from build123d import *

# Parameters (mm, degrees)
ESBO_O2_W                = 30
ESBO_O2_H                = 70
RESSALTO_EXTRUS_O1_DEPTH = 8
ESBO_O3_R                = 0.75
CORTE_EXTRUS_O1_DEPTH    = 30
FILETE1_R                = 2
ESBO_O17_W               = 10
ESBO_O17_H               = 5
RESSALTO_EXTRUS_O4_DEPTH = 8
ESBO_O20_R               = 2
CORTE_EXTRUS_O9_DEPTH    = 8
FILETE2_R                = 2.5
FILETE3_R                = 2.5
FILETE4_R                = 2.5
FILETE5_R                = 2.5
ESBO_O21_W               = 5
ESBO_O21_H               = 20
CORTE_EXTRUS_O10_DEPTH   = 9
FILETE6_R                = 2.5
ESBO_O22_R               = 1.5
CORTE_EXTRUS_O11_DEPTH   = 20
ESBO_O23_R               = 1.75
CORTE_EXTRUS_O12_DEPTH   = 22


with BuildPart() as part:
    # Esboço2 → Ressalto-extrusão1 (new body)
    with BuildSketch(Plane.XY):
        with Locations((-52.281248797, -0.107598663)):
            Rectangle(ESBO_O2_W, ESBO_O2_H)
    extrude(amount=RESSALTO_EXTRUS_O1_DEPTH)

    # Esboço3 → Corte-extrusão1 (cut)
    with BuildSketch(Plane(origin=(0, -35.107598663, 0), x_dir=(-1, 0, 0), z_dir=(0, -1, 0))):
        with Locations((58.281248797, -4)):
            Circle(ESBO_O3_R)
        with Locations((63.281248797, -4)):
            Circle(ESBO_O3_R)
    extrude(amount=-CORTE_EXTRUS_O1_DEPTH, mode=Mode.SUBTRACT)

    # Filete1
    filete1_edges = [part.edges().sort_by_distance(p)[0] for p in [
        (-37.281248797, -0.107598663, 8),
    ]]
    fillet(filete1_edges, radius=FILETE1_R)

    # Esboço17 → Ressalto-extrusão4 (add)
    with BuildSketch(Plane(origin=(0, 0, 0), x_dir=(-1, 0, 0), z_dir=(0, 0, -1))):
        with Locations((72.281248797, -32.607598663)):
            Rectangle(ESBO_O17_W, ESBO_O17_H)
    extrude(amount=-RESSALTO_EXTRUS_O4_DEPTH)

    # Esboço20 → Corte-extrusão9 (cut)
    with BuildSketch(Plane.XZ.offset(35.107598663)):
        with Locations((-73.951248797, 4)):
            Circle(ESBO_O20_R)
    extrude(amount=-CORTE_EXTRUS_O9_DEPTH, mode=Mode.SUBTRACT)

    # Filete2
    filete2_edges = [part.edges().sort_by_distance(p)[0] for p in [
        (-67.281248797, 2.392401337, 8),
    ]]
    fillet(filete2_edges, radius=FILETE2_R)

    # Filete3
    filete3_edges = [part.edges().sort_by_distance(p)[0] for p in [
        (-67.281248797, 2.392401337, 0),
    ]]
    fillet(filete3_edges, radius=FILETE3_R)

    # Filete4
    filete4_edges = [part.edges().sort_by_distance(p)[0] for p in [
        (-77.281248797, -32.607598663, 8),
    ]]
    fillet(filete4_edges, radius=FILETE4_R)

    # Filete5
    filete5_edges = [part.edges().sort_by_distance(p)[0] for p in [
        (-77.281248797, -32.607598663, 0),
    ]]
    fillet(filete5_edges, radius=FILETE5_R)

    # Esboço21 → Corte-extrusão10 (cut, through all)
    with BuildSketch(Plane.XY.offset(8)):
        with Locations((-44.781248797, 18.892401337)):
            Rectangle(ESBO_O21_W, ESBO_O21_H)
        with Locations((-44.781248797, -19.107598663)):
            Rectangle(ESBO_O21_W, ESBO_O21_H)
    extrude(amount=-CORTE_EXTRUS_O10_DEPTH, mode=Mode.SUBTRACT)

    # Filete6
    filete6_edges = [part.edges().sort_by_distance(p)[0] for p in [
        (-37.281248797, -0.107598663, 0),
    ]]
    fillet(filete6_edges, radius=FILETE6_R)

    # Esboço22 → Corte-extrusão11 (cut)
    with BuildSketch(Plane(origin=(-37.281248797, 0, 0), x_dir=(0, 0, -1), z_dir=(1, 0, 0))):
        with Locations((-5, -25.107598663)):
            Circle(ESBO_O22_R)
        with Locations((-5, -14.107598663)):
            Circle(ESBO_O22_R)
        with Locations((-5, 24.892401337)):
            Circle(ESBO_O22_R)
        with Locations((-5, 13.892401337)):
            Circle(ESBO_O22_R)
    extrude(amount=-CORTE_EXTRUS_O11_DEPTH, mode=Mode.SUBTRACT)

    # Esboço23 → Corte-extrusão12 (cut)
    with BuildSketch(Plane(origin=(0, 34.892401337, 0), x_dir=(1, 0, 0), z_dir=(0, 1, 0))):
        with Locations((-62.281248797, -4)):
            Circle(ESBO_O23_R)
    extrude(amount=-CORTE_EXTRUS_O12_DEPTH, mode=Mode.SUBTRACT)


solid = part.part
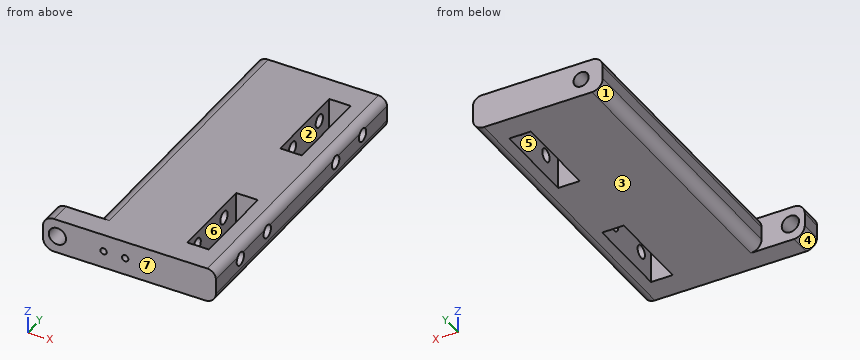
Read the model definition and answer for the solid it produces. Units are mm, in the model's axes. Face numbers are marked on the shaded views. A direction names the side the tool comes from. Round coordinates to 2 decimals unless told otherwise and drop trailing zeros. Order: outer loops, then holes, each group sorted by start corner. A loop starts at its lowest first (then second) coordinate and runs counter-clockwise, first axis right, second up. Notation, with made-up numbers: (-7.5, -19.5) - (7.5, -19.5) arc R31 ccw to (7.5, 13.5) - close; hole circle Ø9 at (54, 55). An arc over 180 degrees is marked (long way). Use one line per item in the form item = value. Start each with the question number.
(1) Flat-ended cylindrical pins translate along their axes: pin 1 Ø1 at (y, z) = (-4.5, 5.5) entering from -X; pin 2 Ø2.5 at (y, z) = (13.89, 5) entering from +X; pin 3 Ø0.8 at (x, z) = (-63.5, 4) entering from -Y; pin 4 Ø3.5 at (x, z) = (-73.95, 4) entering from -Y. Find the tip coordinate at first contact, or state that the pin passes through.
(2) Determine the mould class of the marked faces 4, 5, 6 and 7 for opening direction Y: +Y half, -Y half, draft (parallel to the pull), parting line (faces both ways), or undercut.
(3) The part is cut by section C-C (z = 1.25). Give the vertices of the cut face in (x, y).
(4) The part is cut by section A-A (y = -17). Give the vertices of the cut face in (x, z).
(5) Find the intervals of material crossed by line 1 along X through (y, z) = (-22.75, 4); line 2 along Y through (x, z) = (-39.3, 5); line 3 along Z through (x, y) = (-62.5, 26), in increasing order. Write a range as from..to.
(6) For the marked faces 1, 2 and 3, determine the directions among +Z, -Z, +X, -X, +Y, -Y from which every point of the face is accessible in a straight line to the end or side of a thin tool.
(7) The part is cut by section B-B (y = 11.5). Give the vertices of the cut face in (x, z).
Checked values:
q1.pin_1 = -67.28
q1.pin_2 = -57.28
q1.pin_3 = -5.11
q1.pin_4 = through
q2.face_4 = draft
q2.face_5 = undercut
q2.face_6 = undercut
q2.face_7 = -Y half
q3.outline = (-76.95, -35.11) - (-37.62, -35.11) - (-37.62, 34.89) - (-66.95, 34.89) - (-66.95, -30.11) - (-76.95, -30.11) - close; hole (-47.28, -29.11) - (-42.28, -29.11) - (-42.28, -9.11) - (-47.28, -9.11) - close; hole (-47.28, 8.89) - (-42.28, 8.89) - (-42.28, 28.89) - (-47.28, 28.89) - close
q4.outline = (-67.28, 2.5) arc R2.5 ccw to (-64.78, 0) - (-47.28, 0) - (-47.28, 8) - (-64.78, 8) arc R2.5 ccw to (-67.28, 5.5) - close; (-42.28, 0) - (-39.78, 0) arc R2.5 ccw to (-37.28, 2.5) - (-37.28, 6) arc R2 ccw to (-39.28, 8) - (-42.28, 8) - close; hole circle Ø1.5 at (-63.28, 4); hole circle Ø1.5 at (-58.28, 4)
q5.line_1 = -67.28..-64.03, -62.53..-59.03, -57.53..-47.28, -42.28..-37.28
q5.line_2 = -35.11..-26.61, -23.61..-15.61, -12.61..12.39, 15.39..23.39, 26.39..34.89
q5.line_3 = 0..2.26, 5.74..8
q6.face_1 = -Z, -X, +Y
q6.face_2 = +Z, -Z
q6.face_3 = -Z, +X, -X, +Y, -Y
q7.outline = (-67.28, 2.5) arc R2.5 ccw to (-64.78, 0) - (-47.28, 0) - (-47.28, 8) - (-64.78, 8) arc R2.5 ccw to (-67.28, 5.5) - close; (-42.28, 0) - (-39.78, 0) arc R2.5 ccw to (-37.28, 2.5) - (-37.28, 6) arc R2 ccw to (-39.28, 8) - (-42.28, 8) - close
